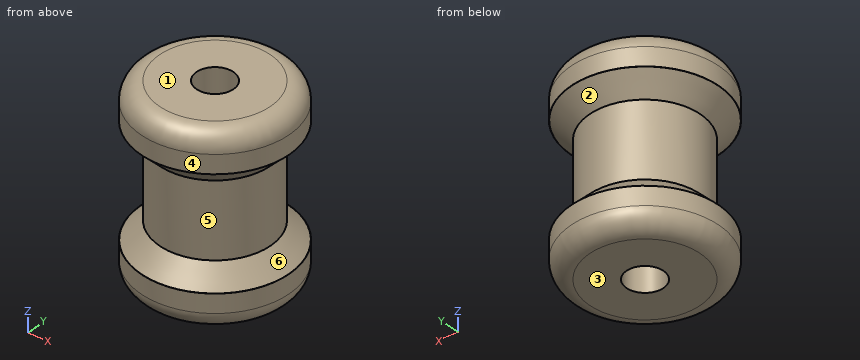
from build123d import *

# Parameters (mm, degrees)
SKETCH_R     = 4
PAD_DEPTH    = 2
SKETCH001_R  = 3
PAD001_DEPTH = 6
SKETCH002_R  = 4
PAD002_DEPTH = 2
SKETCH003_R  = 1
POCKET_DEPTH = 10
CHAMFER_SIZE = 0.99
FILLET_R     = 1


with BuildPart() as part:
    # Sketch → Pad (new body)
    with BuildSketch(Plane.XY):
        Circle(SKETCH_R)
    extrude(amount=PAD_DEPTH)

    # Sketch001 (on Face3 of Pad) → Pad001 (join)
    with BuildSketch(Plane.XY.offset(2)):
        Circle(SKETCH001_R)
    extrude(amount=PAD001_DEPTH)

    # Sketch002 (on Face5 of Pad001) → Pad002 (join)
    with BuildSketch(Plane.XY.offset(8)):
        Circle(SKETCH002_R)
    extrude(amount=PAD002_DEPTH)

    # Sketch003 (on Face3 of Pad002) → Pocket (cut)
    with BuildSketch(Plane.XY.offset(10)):
        Circle(SKETCH003_R)
    extrude(amount=-POCKET_DEPTH, mode=Mode.SUBTRACT)

    # Chamfer
    chamfer_edges = [part.edges().sort_by_distance(p)[0] for p in [
        (-3, 0, 8),
        (-3, 0, 2),
    ]]
    chamfer(chamfer_edges, length=CHAMFER_SIZE)

    # Fillet
    fillet_edges = [part.edges().sort_by_distance(p)[0] for p in [
        (-4, 0, 0),
        (-4, 0, 10),
    ]]
    fillet(fillet_edges, radius=FILLET_R)


solid = part.part
Input: part model. Units: mm. Frame: model coordinates. Face numbers are marked on the shaded views. A direction names the side the tool comes from. Give positions to 0.01 mm unless a question says otherwise; leave off trailing zeros. Write each loop counter-clockwise with the first axis right and the second up, starting at its lowest first coordinate (ties: lowest second). Pieces come first, ordered by that corner, then holes.
Q1. Pull-direction query (Z, two-part tool) for the marked faces 3, 4, 5 and 6; classes: pulls with the +Z half, pulls with the -Z half, needs draft (parallel to the pull), parting line crosses it, or undercut.
Q2. Set-up query: the marked faces 1 and 2. Return all of +Z, -Z, +X, -X, +Y, -Y with unobstructed straight access to the full face (end or side cutting, diameter ignored); none if empty.
Q3. Section C-C, the plane z = 6. Output: boundary loops of the cut face in (x, y), plus the area to 3 significant figures.
Q4. Material intervals for probe 1 along Y at (x, z) = (0, 4.5); probe 2 along Z at (x, y) = (-0.25, 3.75); probe 3 along Y at (x, z) = (0, 0.75), sorted ascending.
Q5. First-contact query: P1, Ø1, axis at x = -3, z = 8.5, coming from the +Y side; P2, Ø1.8, axis at x = 0, y = 0, coming from the +Z side; P3, Ø1, axis at y = 1, z = 3.5, coming from the +X side; P4, Ø2, axis at y = 2, z = 2, coming from the +X side. Flat tips, straight axial feed; report the tip coordinate or a pass-through.
Q6. Section D-D, the plane z = 7.5. Output: boundary loops of the cut face in (x, y), plus the area to 3 significant figures.
Filled in:
1. face 3: pulls with the -Z half
1. face 4: needs draft
1. face 5: undercut
1. face 6: undercut
2. face 1: +Z, +X, -X, +Y, -Y
2. face 2: none
3. outline: circle Ø6 at (0, 0); hole circle Ø2 at (0, 0)
3. area: 25.1 mm2
4. probe 1: y = -3 to -1, 1 to 3
4. probe 2: z = 0.35 to 2.23, 7.77 to 9.65
4. probe 3: y = -3.97 to -1, 1 to 3.97
5. P1: stops at y = 3.12
5. P2: passes through
5. P3: stops at x = 2.96
5. P4: stops at x = 3.87
6. outline: circle Ø6.98 at (0, 0); hole circle Ø2 at (0, 0)
6. area: 35.1 mm2
